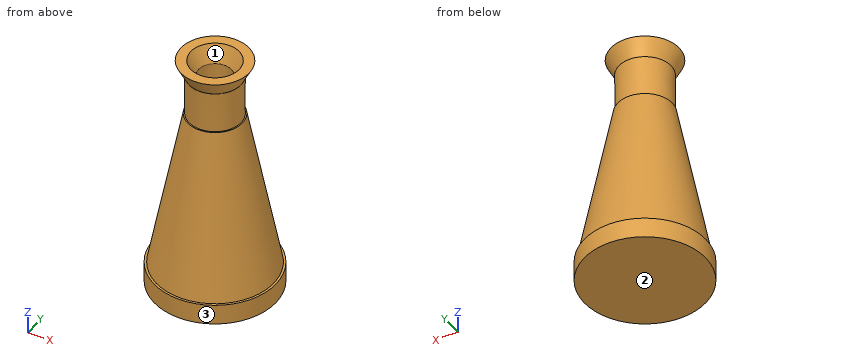
```python
from build123d import *

# Parameters (mm, degrees)
F0_R     = 15
F1_DEPTH = 5


with BuildPart() as f1:
    # F0 (on Top) → F1 (new body)
    with BuildSketch(Plane.XY):
        Circle(F0_R)
    extrude(amount=F1_DEPTH)

    # F2 (on Front) → F3 (revolve)
    with BuildSketch(Plane.XZ):
        Polygon((-14.491172, 4.864085), (0, 4.864085), (0, 44.864085), (-6.733272, 44.864085), align=None)
    revolve(axis=Axis((0, 0, 24.864085), (0, 0, 1)))

    # F4 (on Front) → F5 (revolve)
    with BuildSketch(Plane.XZ):
        Polygon((-6.417496, 44.807569), (0, 44.983736), (0, 54.983736), (-6.434252, 54.983736), align=None)
    revolve(axis=Axis((0, 0, 49.983736), (0, 0, 1)))

    # F6 (on Front) → F7 (revolve)
    with BuildSketch(Plane.XZ):
        Polygon((-8.426686, 58.967727), (-6.387146, 54.967727), (0, 54.967727), (0, 58.967727), align=None)
    revolve(axis=Axis((0, 0, 56.967727), (0, 0, -1)))

    # F8 (on Front) → F9 (revolve, cut)
    with BuildSketch(Plane.XZ):
        Polygon((-4.05009, 44.66689), (-11.844673, 5.362289), (0, 5.528131), (0, 59.371449), (-6.179371, 59.371449), (-4.05009, 54.949105), align=None)
    revolve(axis=Axis((0, 0, 32.44979), (0, 0, -1)), mode=Mode.SUBTRACT)


solid = f1.part
```
The model under review builds one solid part; all positions refer to its coordinate system, in mm. Face numbers are marked on the shaded views. Coordinates: 2 decimals unless noted, no trailing zeros. Write each loop counter-clockwise with the first axis right and the second up, starting at its lowest first coordinate (ties: lowest second). Pieces come first, ordered by that corner, then holes. Notation, with made-up numbers: (-9.5, -22.75) - (42.5, -22.75) arc R29 ccw to (42.5, 3.25) - close; hole circle Ø8 at (9, 76). An arc over 180 degrees is marked (long way). Answer in a Markdown table with one row per item. Add a question column.
Q1. Draft analysis for pull direction Y (two halves, no side actions). For the marked faces 1, 2 and 3, state which applies: +Y half, -Y half, draft (parallel to the pull), parting line (faces both ways), or undercut.
Q2. Clearance check with flat-ended pins moving along their axes: pin 1 (12 mm diameter, centred on x = -11.5, y = -1.5, fed in from +Z); pin 2 (12 mm diameter, centred on x = -3.5, z = 26.5, fed in from +Y); pin 3 (4 mm diameter, centred on x = 1, y = -1.5, fed in from +Z); pin 4 (1 mm diameter, centred on y = 3, z = 40.5, fed in from -X). State where each tip first meets the part, or that it passes through.
Q3. Consider section D-D on z = 38.5. Give the boundary of the cut face in (x, y), then the cut area to 3 significant figures.
Q4. Consider section C-C on z = 22.5. Give the boundary of the cut face in (x, y), then the cut area to 3 significant figures.
Q5. Consider section A-A on x = -7.5. Give the number of separate pieces and of enclosed holes in the cut face, then the cut area to 3 significant figures.
Q6. To check wall thickness, follow line 1 along X through (y, z) = (0, 49); line 2 along Y through (x, z) = (0, 44.8). State the ranges of each line that lie inside material, in increasing order. Write a range as from..to.
Answers below:
| question | item | result |
|---|---|---|
| 1 | face 1 | undercut |
| 1 | face 2 | draft |
| 1 | face 3 | parting line |
| 2 | pin 1 | z = 58.97 |
| 2 | pin 2 | y = 11.31 |
| 2 | pin 3 | z = 5.53 |
| 2 | pin 4 | x = -7.18 |
| 3 | outline | circle Ø15.94 at (0, 0); hole circle Ø10.55 at (0, 0) |
| 3 | area | 112 mm² |
| 4 | outline | circle Ø22.14 at (0, 0); hole circle Ø16.89 at (0, 0) |
| 4 | area | 161 mm² |
| 5 | separate pieces | 2 |
| 5 | enclosed holes | 1 |
| 5 | area | 437 mm² |
| 6 | line 1 | -6.42..-4.05, 4.05..6.42 |
| 6 | line 2 | -6.75..-4.05, 4.05..6.75 |
